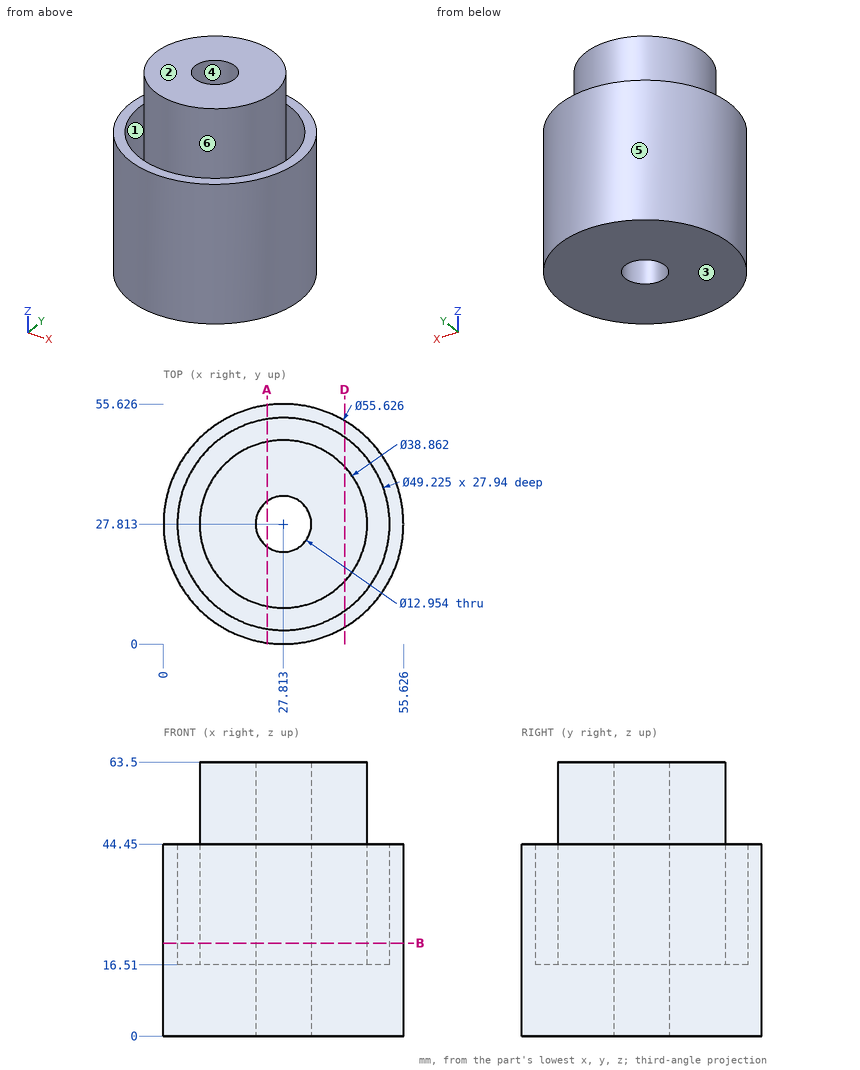
Geometry: see drawing. Coordinates: mm, zero at the bounding-box minimum. A direction names the side the tool comes from. Give positions to 0.01 mm unless a question says otherwise; leave off trailing zeros. Order: outer loops, then holes, each group sorted by start corner. A loop starts at its lowest first (then second) coordinate and runs counter-clockwise, first axis right, second up.
Q1. Contact query for flat-ended pins moving along their axis: pin 1 Ø8 at (y, z) = (20.5, 16) entering from +X; pin 2 Ø1.5 at (x, z) = (24.5, 35) entering from -Y; pin 3 Ø3 at (y, z) = (31, 13.5) entering from -X; pin 4 Ø11.5 at (x, y) = (27.813, 27.813) entering from +Z. Output: stop coordinate, or through.
Checked values:
pin 1: stops at x = 55.43
pin 2: stops at y = 0.12
pin 3: stops at x = 0.05
pin 4: passes through
Q2. Section A-A on x = 24. Output: boundary loops of the cut face in (y, z).
Checked values:
outline: (0.26, 0) - (22.58, 0) - (22.58, 63.5) - (8.76, 63.5) - (8.76, 16.51) - (3.5, 16.51) - (3.5, 44.45) - (0.26, 44.45) - close; (33.05, 0) - (55.36, 0) - (55.36, 44.45) - (52.13, 44.45) - (52.13, 16.51) - (46.87, 16.51) - (46.87, 63.5) - (33.05, 63.5) - close
Q3. Section D-D on x = 42. Output: boundary loops of the cut face in (y, z).
Checked values:
outline: (3.89, 0) - (51.74, 0) - (51.74, 44.45) - (47.93, 44.45) - (47.93, 16.51) - (41.09, 16.51) - (41.09, 63.5) - (14.54, 63.5) - (14.54, 16.51) - (7.7, 16.51) - (7.7, 44.45) - (3.89, 44.45) - close
Q4. Ray query, probe 1 along Y at (x, z) = (27.5, 59.5); probe 2 along Y at (x, z) = (28.5, 27); probe 3 along Y at (x, z) = (29, 22.5) (1 decimal). Return the intervals inside material, ascending.
Checked values:
probe 1: y = 8.38 to 21.34, 34.28 to 47.24
probe 2: y = 0.01 to 3.21, 8.39 to 21.37, 34.25 to 47.23, 52.42 to 55.62
probe 3: y = 0 to 3.2, 8.4 to 21.4, 34.2 to 47.2, 52.4 to 55.6
Q5. Section B-B on z = 21.5. Output: boundary loops of the cut face in (x, y) (1 decimal), and give its area (3 significant figures).
Checked values:
outline: circle Ø55.6 at (27.8, 27.8); circle Ø38.9 at (27.8, 27.8); hole circle Ø49.2 at (27.8, 27.8); hole circle Ø13 at (27.8, 27.8)
area: 1,580 mm2
Q6. Draft query along X for the marked faces 3, 4, 5 and 6. Return one class per face: +X half, -X half, draft (parallel to the pull), parting line (faces both ways), or undercut.
Checked values:
face 3: draft
face 4: undercut
face 5: parting line
face 6: undercut
Q7. Set-up query: the marked faces 1 and 2. Return all of +Z, -Z, +X, -X, +Y, -Y with unobstructed straight access to the full face (end or side cutting, diameter ignored); none if empty.
Checked values:
face 1: +Z
face 2: +Z, +X, -X, +Y, -Y
